The model under review builds one solid part; all positions refer to its coordinate system, in mm. Face numbers are marked on the shaded views. Round coordinates to 2 decimals unless told otherwise and drop trailing zeros. Write each loop counter-clockwise with the first axis right and the second up, starting at its lowest first coordinate (ties: lowest second). Pieces come first, ordered by that corner, then holes. Notation, with made-up numbers: (-14.75, 12.5) - (20.25, 12.5) arc R33 cw to (20.25, 50.5) - close; hole circle Ø10 at (77.5, -9.5). An arc over 180 degrees is marked (long way). One line per question, with ' | ' between items. Start each with the question number.
```python
from build123d import *

# Parameters (mm, degrees)
ESBO_O1_W                = 38.5
ESBO_O1_H                = 34
RESSALTO_EXTRUS_O1_DEPTH = 2.5
ESBO_O2_W                = 2.5
ESBO_O2_H                = 6
ESBO_O2_H_2              = 5.5
RESSALTO_EXTRUS_O2_DEPTH = 12.5
CORTE_EXTRUS_O1_REACH    = 42.236
ESBO_O3_R                = 1.5
ESBO_O4_W                = 2.95
ESBO_O4_H                = 20
RESSALTO_EXTRUS_O3_DEPTH = 13
ESBO_O5_R                = 3.45
CORTE_EXTRUS_O2_DEPTH    = 15
FILETE1_R                = 3
FILETE2_R                = 2.5
ESBO_O7_R                = 3.45
RESSALTO_EXTRUS_O5_DEPTH = 6
ESBO_O8_R                = 1.6
CORTE_EXTRUS_O3_DEPTH    = 6
FILETE3_R                = 2
FILETE4_R                = 5
FILETE5_R                = 2


with BuildPart() as part:
    # Esboço1 → Ressalto-extrusão1 (new body)
    with BuildSketch(Plane.XY):
        with Locations((-3.395014232, -10.289862205)):
            Rectangle(ESBO_O1_W, ESBO_O1_H)
    extrude(amount=RESSALTO_EXTRUS_O1_DEPTH)

    # Esboço2 → Ressalto-extrusão2 (add)
    with BuildSketch(Plane.XY.offset(2.5)):
        with Locations((1.584985768, 3.710137795)):
            Rectangle(ESBO_O2_W, ESBO_O2_H)
        with Locations((1.584985768, -24.539862205)):
            Rectangle(ESBO_O2_W, ESBO_O2_H_2)
    extrude(amount=RESSALTO_EXTRUS_O2_DEPTH)

    # Esboço3 → Corte-extrusão1 (cut, up to next)
    with BuildSketch(Plane(origin=(2.834985768, 0, 0), x_dir=(0, 0, -1), z_dir=(1, 0, 0)), mode=Mode.PRIVATE) as corte_extrus_o1_sk1:
        with Locations(Location((-11.5, 3.410137795, 0), (0, 0, 90))):
            Circle(ESBO_O3_R)
    corte_extrus_o1_tool1 = extrude(corte_extrus_o1_sk1.sketch, amount=-CORTE_EXTRUS_O1_REACH, mode=Mode.PRIVATE) & part.part
    # Esboço3 → Corte-extrusão1 (cut, up to next)
    with BuildSketch(Plane(origin=(2.834985768, 0, 0), x_dir=(0, 0, -1), z_dir=(1, 0, 0)), mode=Mode.PRIVATE) as corte_extrus_o1_sk2:
        with Locations(Location((-11.5, -23.789862205, 0), (0, 0, 90))):
            Circle(ESBO_O3_R)
    corte_extrus_o1_tool2 = extrude(corte_extrus_o1_sk2.sketch, amount=-CORTE_EXTRUS_O1_REACH, mode=Mode.PRIVATE) & part.part
    add(corte_extrus_o1_tool1.solids().sort_by_distance((2.834986, 3.410138, 11.5))[0], mode=Mode.SUBTRACT)
    add(corte_extrus_o1_tool2.solids().sort_by_distance((2.834986, -23.789862, 11.5))[0], mode=Mode.SUBTRACT)

    # Esboço4 → Ressalto-extrusão3 (add)
    with BuildSketch(Plane.XY.offset(2.5)):
        with Locations((-21.170014232, -17.289862205)):
            Rectangle(ESBO_O4_W, ESBO_O4_H)
    extrude(amount=RESSALTO_EXTRUS_O3_DEPTH)

    # Esboço5 → Corte-extrusão2 (cut)
    with BuildSketch(Plane.ZY.offset(22.645014232)):
        Polygon((2.5, -7.289862205), (15.222036194, -11.595443281), (15.5, -11.689515935), (15.5, -7.289862205), align=None)
        Polygon((15.222036194, -16.59994967), (2.5, -27.289862205), (15.5, -27.289862205), (15.5, -16.36638574), align=None)
        with Locations(Location((9.45, -15.089862205, 0), (0, 0, 270))):
            Circle(ESBO_O5_R)
    extrude(amount=-CORTE_EXTRUS_O2_DEPTH, mode=Mode.SUBTRACT)

    # Filete1
    filete1_edges = [part.edges().sort_by_distance(p)[0] for p in [
        (-21.170014232, -11.689515935, 15.5),
        (-21.170014232, -16.36638574, 15.5),
    ]]
    fillet(filete1_edges, radius=FILETE1_R)

    # Filete2
    # the kernel refuses this fillet: 2.5 mm, written as the material it adds along each edge
    with BuildSketch(Plane(origin=(-19.695014232, -7.289862205, 2.5), x_dir=(0, -0.32057353707536407, 0.947223631106715), z_dir=(-1, 0, 0))) as filete2_piece_1:
        with BuildLine():
            CenterArc((FILETE2_R * 0.717282002488, FILETE2_R), FILETE2_R, 198.697613514, 71.302386486)
            Line((-FILETE2_R * 0.229941628618, FILETE2_R * 0.679426462925), (0, 0))
            Line((0, 0), (FILETE2_R * 0.717282002488, 0))
        make_face()
    extrude(amount=2.95)

    # Esboço7 → Ressalto-extrusão5 (add)
    with BuildSketch(Plane.ZY.offset(22.645014232)):
        with Locations(Location((9.45, -15.089862205, 0), (0, 0, 270))):
            Circle(ESBO_O7_R)
    extrude(amount=-RESSALTO_EXTRUS_O5_DEPTH)

    # Esboço8 → Corte-extrusão3 (cut)
    with BuildSketch(Plane(origin=(0, 0, 0), x_dir=(-1, 0, 0), z_dir=(0, 0, -1))):
        with Locations((7.965014232, -19.289862205)):
            Circle(ESBO_O8_R)
        with Locations((-6.754985768, -14.739862205)):
            Circle(ESBO_O8_R)
    extrude(amount=-CORTE_EXTRUS_O3_DEPTH, mode=Mode.SUBTRACT)

    # Filete3
    filete3_edges = [part.edges().sort_by_distance(p)[0] for p in [
        (1.584985768, -21.789862205, 2.5),
        (1.584985768, 0.710137795, 2.5),
    ]]
    fillet(filete3_edges, radius=FILETE3_R)

    # Filete4
    filete4_edges = [part.edges().sort_by_distance(p)[0] for p in [
        (1.584985768, -27.289862205, 15),
        (1.584985768, 6.710137795, 15),
    ]]
    fillet(filete4_edges, radius=FILETE4_R)

    # Filete5
    filete5_edges = [part.edges().sort_by_distance(p)[0] for p in [
        (1.584985768, 0.710137795, 15),
        (1.584985768, -21.789862205, 15),
    ]]
    fillet(filete5_edges, radius=FILETE5_R)


solid = part.part
```
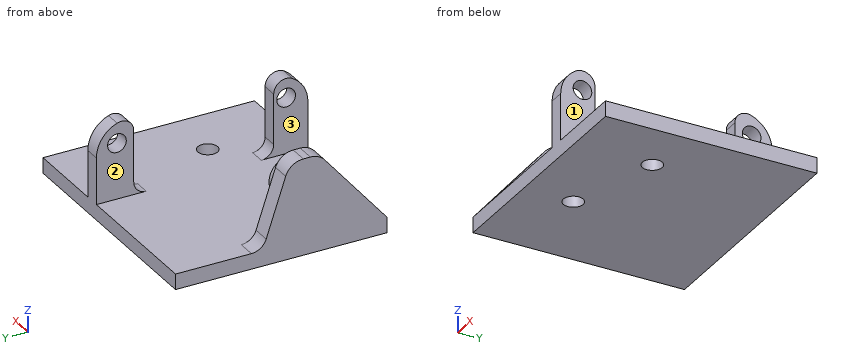
1. The part is to be moulded in two halves that separate along X. For the marked faces 1, 2 and 3, say which applies: pulls with the +X half, pulls with the -X half, needs draft (parallel to the pull), parting line crosses it, or undercut.
2. Add section B-B, the plane x = 6. Write out the cut boundary in (y, z), then the cut area to 3 significant figures.
3. Add section C-C, the plane z = 11.5. Write out the cut boundary in (x, y), then the cut area to 3 significant figures.
4. Wall thickness on line 1 along Y through (x, z) = (1, 9.5); line 2 along Z through (x, y) = (-1.5, -24); line 3 along X through (y, z) = (-11, 10): over which ranges is each line inside the solid? List them lowest first. Write a range as [from, to].
5. Clearance check with flat-ended pins moving along their axes: P1, Ø6.5, axis at y = 3.5, z = 9.5, coming from the -X side (3 decimals); P2, Ø5.5, axis at y = -15.5, z = 11, coming from the +X side (3 decimals); P3, Ø1.5, axis at x = -14.5, y = -14, coming from the +Z side. State where each tip first meets the part, or that it passes through.
6. Add section D-D, the plane y = -2. Write out the cut boundary in (x, z).
7. Add section A-A, the plane z = 9. Write out the cut boundary in (x, y).
Geometry check:
1) face 1: pulls with the +X half | face 2: pulls with the -X half | face 3: undercut
2) outline: (-27.29, 0) - (-16.15, 0) - (-16.15, 2.5) - (-27.29, 2.5) - close; (-13.33, 0) - (6.71, 0) - (6.71, 2.5) - (-13.33, 2.5) - close | area: 77.9 mm2
3) outline: (-22.65, -19.73) - (-19.7, -19.73) - (-19.7, -17.86) - (-16.65, -17.86) - (-16.65, -12.31) - (-19.7, -12.31) - (-19.7, -10.34) - (-22.65, -10.34) - close; (0.33, -27.06) - (2.83, -27.06) - (2.83, -25.29) - (0.33, -25.29) - close; (0.33, -22.29) - (2.83, -22.29) - (2.83, -21.79) - (0.33, -21.79) - close; (0.33, 0.71) - (2.83, 0.71) - (2.83, 1.91) - (0.33, 1.91) - close; (0.33, 4.91) - (2.83, 4.91) - (2.83, 6.48) - (0.33, 6.48) - close | area: 57.2 mm2
4) line 1: y = [-27.29, -21.79], [0.71, 6.71] | line 2: z = [0, 2.5] | line 3: x = [-22.65, -19.7]
5) P1: stops at x = 0.335 | P2: stops at x = -16.645 | P3: stops at z = 2.5
6) outline: (-22.65, 0) - (15.85, 0) - (15.85, 2.5) - (-22.65, 2.5) - close
7) outline: (-22.65, -21.83) - (-19.7, -21.83) - (-19.7, -18.51) - (-16.65, -18.51) - (-16.65, -11.67) - (-19.7, -11.67) - (-19.7, -9.49) - (-22.65, -9.49) - close; (0.33, -27.29) - (2.83, -27.29) - (2.83, -21.79) - (0.33, -21.79) - close; (0.33, 0.71) - (2.83, 0.71) - (2.83, 6.71) - (0.33, 6.71) - close
